Input: dimensioned drawing with shaded views. Units: mm. Origin: part minimum x, y, z. Round coordinates to 2 decimals unless told otherwise and drop trailing zeros. Order: outer loops, then holes, each group sorted by start corner. A loop starts at its lowest first (then second) coordinate and runs counter-clockwise, first axis right, second up.
Item 1: Line query: L1, parallel to Y at x = 15, z = 0.9; L2, parallel to Y at x = 15, z = 2.55. Output: solid intervals per line, ascending.
Item 2: Cut plane B-B on y = 15. Output: boundary loops of the cut face in (x, z).
Item 3: Cut plane C-C on z = 1.85. Output: boundary loops of the cut face in (x, y), then the cut area to 3 significant figures.
Item 4: Mould query, pull axis X, two halves, no side actions, for the marked faces 1, 2 and 3. Classes: released by +X, released by -X, zero draft, split by the parting line, or undercut.
Item 5: First-contact query: pin 1 (1.5 mm diameter, centred on x = 13.5, z = 2, fed in from -Y); pin 2 (1.2 mm diameter, centred on y = 16, z = 4, fed in from +X); pin 3 (1 mm diameter, centred on x = 15.5, z = 1, fed in from +Y); pin 4 (1 mm diameter, centred on x = 17.5, z = 3, fed in from +Y). Flat tips, straight axial feed; report the tip coordinate or a pass-through.
Item 6: Cut plane A-A on x = 15. Output: boundary loops of the cut face in (y, z), then the cut area to 3 significant figures.
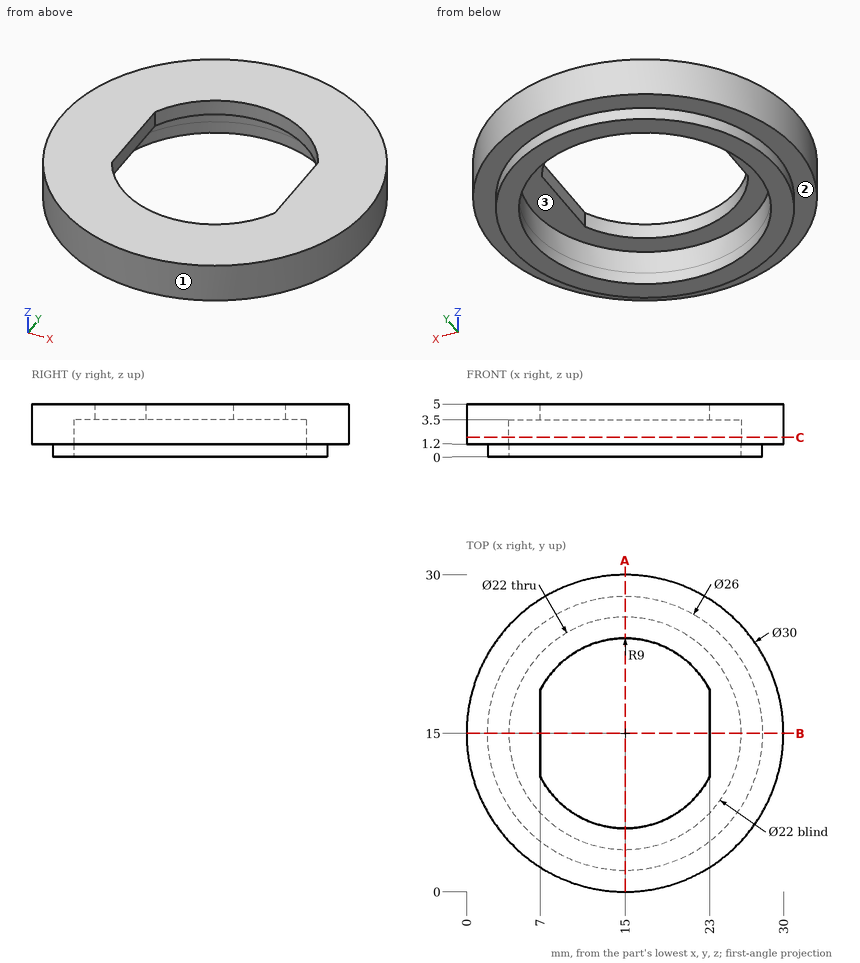
From the geometry:
1. L1: y = 2 to 4, 26 to 28
1. L2: y = 0 to 4, 26 to 30
2. outline: (0, 1.2) - (2, 1.2) - (2, 0) - (4, 0) - (4, 3.5) - (7, 3.5) - (7, 5) - (0, 5) - close; (23, 3.5) - (26, 3.5) - (26, 0) - (28, 0) - (28, 1.2) - (30, 1.2) - (30, 5) - (23, 5) - close
3. outline: circle Ø30 at (15, 15); hole circle Ø22 at (15, 15)
3. area: 327 mm2
4. face 1: split by the parting line
4. face 2: zero draft
4. face 3: undercut
5. pin 1: stops at y = 0.02
5. pin 2: stops at x = 29.99
5. pin 3: stops at y = 30
5. pin 4: stops at y = 29.87
6. outline: (0, 1.2) - (2, 1.2) - (2, 0) - (4, 0) - (4, 3.5) - (6, 3.5) - (6, 5) - (0, 5) - close; (24, 3.5) - (26, 3.5) - (26, 0) - (28, 0) - (28, 1.2) - (30, 1.2) - (30, 5) - (24, 5) - close
6. area: 41.2 mm2
